Autodesk Inventor part; units mm, degrees
ref_plane "YZ Plane" through (0, 0, 0) normal (1, 0, 0) x (0, 1, 0)
ref_plane "XZ Plane" through (0, 0, 0) normal (0, 1, 0) x (-1, 0, 0)
ref_plane "XY Plane" through (0, 0, 0) normal (0, 0, 1) x (1, 0, 0)
sketch "Sketch1" plane through (0, 0, 0) normal (0, 0, 1) x (1, 0, 0)
  circle A0 centre (0, 0) radius 8.255
  circle A1 centre (0, 0) radius 14.859
  dimension "d0" = 16.51
  dimension "d1" = 29.718
extrude "Extrusion1" add sketch "Sketch1" along normal mid plane 1.016
fillet "Fillet1" radius 0.127 1 edges at (-14.859, 0, 0.508)
properties part number "Large Washer" material "Stainless Steel"
Source: CAD feature listing. Evaluate the final solid. Frame: model axes, mm. Coordinates: 2 decimals unless noted, no trailing zeros. Loops run counter-clockwise (first coordinate to the right, second up) from the corner with the lowest first, then second, coordinate; pieces in that order, holes last. Notation, with made-up numbers: M 72.5,60 L 114.5,60 A30 ccw 114.5,96 Z; hole C -18.75,68 d3. An arc over 180 degrees is marked long. Use CSV: the item, a comma, the result in double quotes.
(1) Line query: line 1 (Y direction, x = 0, z = 0.05) (3 decimals); line 2 (Y direction, x = 6.25, z = -0.2); line 3 (X direction, y = -7.5, z = -0.45). Output: solid intervals per line, ascending. Write a range as [from, to].
Answers follow:
line 1,"[-14.859, -8.255], [8.255, 14.859]"
line 2,"[-13.48, -5.39], [5.39, 13.48]"
line 3,"[-12.83, -3.45], [3.45, 12.83]"
(2) Draft query along Y for faces 1 (the face through (7.874, 2.48, 0.007)), 2 (the face through (6, -6, 0.508)), 3 (the face through (-3.221, -14.506, -0.057)). Return one class per face: pulls with the +Y half, pulls with the -Y half, needs draft (parallel to the pull), parting line crosses it, or undercut.
Answers follow:
face 1,"undercut"
face 2,"needs draft"
face 3,"parting line crosses it"
(3) Cut plane A-A on x = 0. Return loops of the section in (y, z) (3 decimals), and give its area (3 significant figures).
Answers follow:
outline,"M -14.859,-0.508 L -8.255,-0.508 L -8.255,0.508 L -14.732,0.508 A0.127 ccw -14.859,0.381 Z; M 8.255,-0.508 L 14.859,-0.508 L 14.859,0.381 A0.127 ccw 14.732,0.508 L 8.255,0.508 Z"
area,"13.4 mm²"
(4) Cut plane C-C on z = -0.15. Return loops of the section in (x, y) (3 decimals), and give its area (3 significant figures).
Answers follow:
outline,"C 0,0 d29.718; hole C 0,0 d16.51"
area,"480 mm²"
